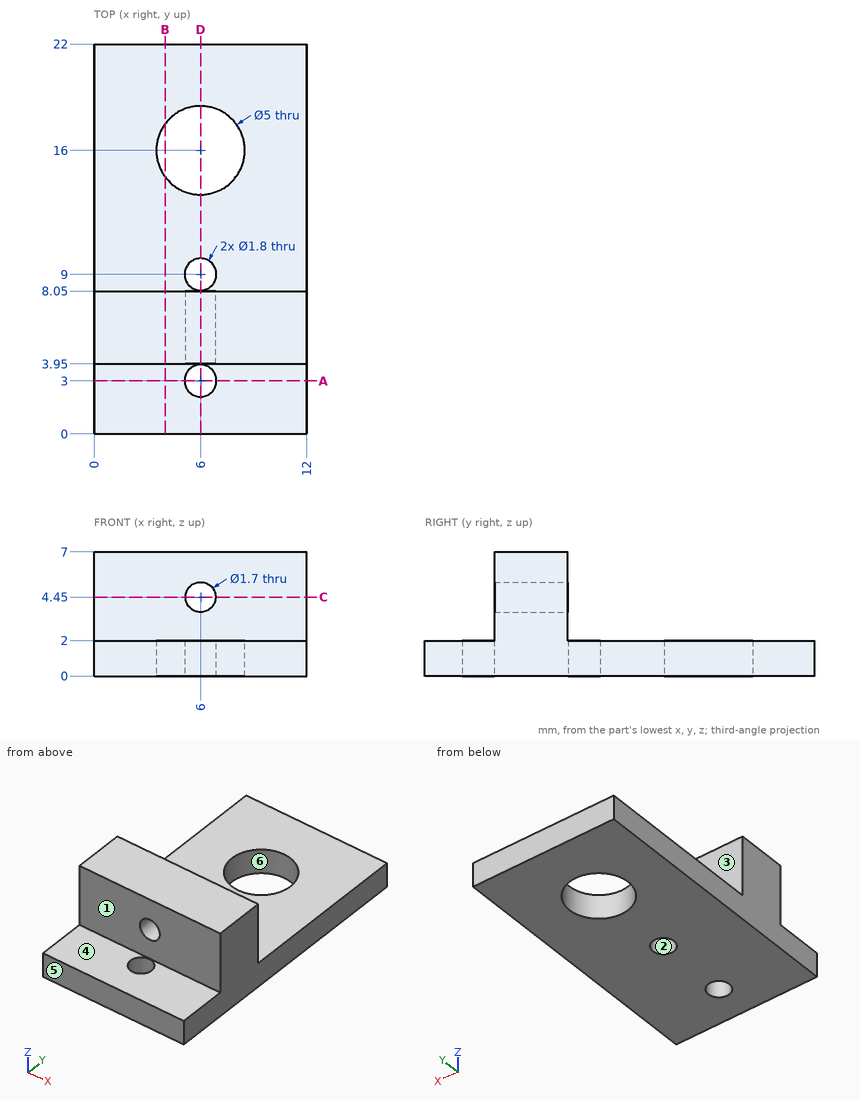
The drawing under review shows one solid part. Ordinate dimensions are in mm from its lowest x, y, z. A direction names the side the tool comes from. Coordinates: 2 decimals unless noted, no trailing zeros. Write each loop counter-clockwise with the first axis right and the second up, starting at its lowest first coordinate (ties: lowest second). Pieces come first, ordered by that corner, then holes. Notation, with made-up numbers: (-5, 6) - (4, 6) arc R31 cw to (4, 42) - close; hole circle Ø10 at (41.25, 36.5). An arc over 180 degrees is marked (long way). Answer as CSV lines item,"result".
(1) We need section A-A (y = 3). Give the boundary of the cut face in (x, z).
Data:
outline,"(0, 0) - (5.1, 0) - (5.1, 2) - (0, 2) - close; (6.9, 0) - (12, 0) - (12, 2) - (6.9, 2) - close"
(2) For line 1 along Y through (x, z) = (6, 0.7); line 2 along Z through (x, y) = (9.5, 1); line 3 along Y through (x, z) = (8.75, 5.5), list the stretches that pass through material, from the lowest coordinate up. Write a range as [from, to].
Data:
line 1,"y = [0, 2.1], [3.9, 8.1], [9.9, 13.5], [18.5, 22]"
line 2,"z = [0, 2]"
line 3,"y = [3.95, 8.05]"
(3) We need section C-C (z = 4.45). Give the boundary of the cut face in (x, y), plus the area to 3 significant figures.
Data:
outline,"(0, 3.95) - (5.15, 3.95) - (5.15, 8.05) - (0, 8.05) - close; (6.85, 3.95) - (12, 3.95) - (12, 8.05) - (6.85, 8.05) - close"
area,"42.2 mm2"
(4) We need section B-B (x = 4). Give the boundary of the cut face in (y, z), plus the area to 3 significant figures.
Data:
outline,"(0, 0) - (14.5, 0) - (14.5, 2) - (8.05, 2) - (8.05, 7) - (3.95, 7) - (3.95, 2) - (0, 2) - close; (17.5, 0) - (22, 0) - (22, 2) - (17.5, 2) - close"
area,"58.5 mm2"
(5) Tool access review of the marked faces 1, 2 and 3: name each direction out of +Z, -Z, +X, -X, +Y, -Y from which nothing blocks a thin tool from reaching the whole face with its end or side.
Data:
face 1,"+Z, +X, -X, -Y"
face 2,"+Z, -Z"
face 3,"+Z, +X, -X, +Y"
(6) Mouldability with a two-part tool opening along Y and no side actions: class the marked faces 4, 5 and 6 as pulls with the +Y half, pulls with the -Y half, needs draft (parallel to the pull), parting line crosses it, or undercut.
Data:
face 4,"needs draft"
face 5,"pulls with the -Y half"
face 6,"undercut"
(7) We need section D-D (x = 6). Give the boundary of the cut face in (y, z), plus the area to 3 significant figures.
Data:
outline,"(0, 0) - (2.1, 0) - (2.1, 2) - (0, 2) - close; (3.9, 0) - (8.1, 0) - (8.1, 2) - (8.05, 2) - (8.05, 3.6) - (3.95, 3.6) - (3.95, 2) - (3.9, 2) - close; (3.95, 5.3) - (8.05, 5.3) - (8.05, 7) - (3.95, 7) - close; (9.9, 0) - (13.5, 0) - (13.5, 2) - (9.9, 2) - close; (18.5, 0) - (22, 0) - (22, 2) - (18.5, 2) - close"
area,"40.3 mm2"
(8) Clearance check with flat-ended pins moving along their axes: pin 1 Ø6 at (x, y) = (6, 16) entering from +Z; pin 2 Ø2.5 at (x, z) = (6, 4) entering from +Y. State where each tip first meets the part, or that it passes through.
Data:
pin 1,"stops at z = 2"
pin 2,"stops at y = 8.05"
